from build123d import *

# Parameters (mm, degrees)
SKETCH1_W                 = 126.873
SKETCH1_H                 = 14.859
BOSS_EXTRUDE1_DEPTH       = 9.398
SKETCH2_W                 = 6.35
SKETCH2_H                 = 13.335
CUT_EXTRUDE1_DEPTH        = 128.658375969
F_5_CLEARANCE_HOLE1_D     = 3.556
F_5_CLEARANCE_HOLE1_DEPTH = 1.524
F_5_CLEARANCE_HOLE2_D     = 3.556
F_5_CLEARANCE_HOLE2_DEPTH = 14.859
F_5_CLEARANCE_HOLE3_D     = 3.556
FILLET1_R                 = 0.635


with BuildPart() as part:
    # Sketch1 → Boss-Extrude1 (new body)
    with BuildSketch(Plane(origin=(-4.699, 0, 0), x_dir=(0, -1, 0), z_dir=(-1, 0, 0))):
        with Locations((-63.4365, -5.9055)):
            Rectangle(SKETCH1_W, SKETCH1_H)
    extrude(amount=-BOSS_EXTRUDE1_DEPTH)

    # Sketch2 → Cut-Extrude1 (cut, through all)
    with BuildSketch(Plane.XZ):
        with Locations((0, -6.6675)):
            Rectangle(SKETCH2_W, SKETCH2_H)
    extrude(amount=-CUT_EXTRUDE1_DEPTH, mode=Mode.SUBTRACT)

    # #5 Clearance Hole1
    with Locations(Plane(origin=(4.699, 0, 0), x_dir=(0, 0, -1), z_dir=(1, 0, 0))):
        with Locations((8.5725, 112.3315), (8.5725, 122.1105), (8.5725, 102.5525), (8.5725, 92.7735), (8.5725, 82.9945), (8.5725, 73.2155), (8.5725, 63.4365), (8.5725, 53.6575), (8.5725, 43.8785), (8.5725, 34.0995), (8.5725, 24.3205), (8.5725, 14.5415), (8.5725, 4.7625)):
            Hole(F_5_CLEARANCE_HOLE1_D / 2, depth=F_5_CLEARANCE_HOLE1_DEPTH)

    # #5 Clearance Hole2
    with Locations(Plane.XY.offset(1.524)):
        with Locations((0, 112.3315), (0, 122.1105), (0, 102.5525), (0, 92.7735), (0, 82.9945), (0, 73.2155), (0, 63.4365), (0, 53.6575), (0, 43.8785), (0, 34.0995), (0, 24.3205), (0, 14.5415), (0, 4.7625)):
            Hole(F_5_CLEARANCE_HOLE2_D / 2, depth=F_5_CLEARANCE_HOLE2_DEPTH)

    # #5 Clearance Hole3 (through all)
    with Locations(Plane(origin=(-3.175, 0, 0), x_dir=(0, 0, -1), z_dir=(1, 0, 0))):
        with Locations((8.5725, 112.3315), (8.5725, 122.1105), (8.5725, 102.5525), (8.5725, 92.7735), (8.5725, 82.9945), (8.5725, 73.2155), (8.5725, 63.4365), (8.5725, 53.6575), (8.5725, 43.8785), (8.5725, 34.0995), (8.5725, 24.3205), (8.5725, 14.5415), (8.5725, 4.7625)):
            Hole(F_5_CLEARANCE_HOLE3_D / 2)

    # Fillet1
    fillet1_edges = [part.edges().sort_by_distance(p)[0] for p in [
        (-3.937, 126.873, -13.335),
        (-3.937, 0, -13.335),
        (3.937, 0, -13.335),
        (3.937, 126.873, -13.335),
    ]]
    fillet(fillet1_edges, radius=FILLET1_R)


solid = part.part
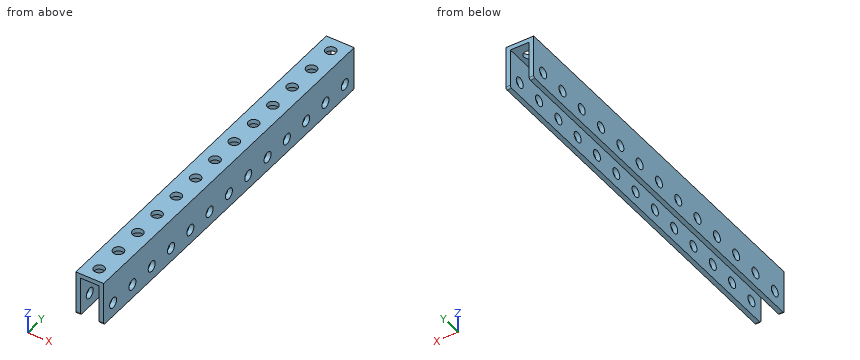
Geometry check sheet. Reference: the model listing, model coordinates, mm. Coordinates: 2 decimals unless noted, no trailing zeros. Order: outer loops, then holes, each group sorted by start corner. A loop starts at its lowest first (then second) coordinate and runs counter-clockwise, first axis right, second up. Notation, with made-up numbers: (79, 24.25) - (102, 24.25) arc R16 ccw to (102, 49.25) - close; hole circle Ø10 at (16.25, -39.5). An arc over 180 degrees is marked (long way). Answer in a Markdown table with one row per item. Add a question column.
1) Cross-section at A-A, the plane y = 49. Record the cut outline in (x, z) (3 decimals), then the cut area to 3 significant figures.
2) Material ranges on line 1 along X through (y, z) = (59, -11.5) (3 decimals); line 2 along Z through (x, y) = (-4, 64.5) (3 decimals); line 3 along Z through (x, y) = (-0.25, 36), recorded low to high. Write a range as [from, to].
3) Cross-section at B-B, the plane x = 0. State how many separate pieces and enclosed holes the cut face has, then the cut area to 3 significant figures.
4) Gauge pin test, flat ends, axial feed: P1, Ø3, axis at x = 0.5, z = -3.5, coming from the -Y side; P2, Ø4, axis at x = 0, y = 53.66, coming from the -Z side. Record the tip position at first contact, or that the pin passes through.
Check result:
| question | item | result |
|---|---|---|
| 1 | outline | (-4.699, -13.335) - (-3.175, -13.335) - (-3.175, 0) - (3.175, 0) - (3.175, -13.335) - (4.699, -13.335) - (4.699, 1.524) - (-4.699, 1.524) - close |
| 1 | area | 55.0 mm² |
| 2 | line 1 | x = [-4.699, -3.175], [3.175, 4.699] |
| 2 | line 2 | z = [-13.335, -9.997], [-7.148, 1.524] |
| 2 | line 3 | z = [0, 1.52] |
| 3 | separate pieces | 14 |
| 3 | enclosed holes | 0 |
| 3 | area | 123 mm² |
| 4 | P1 | passes through |
| 4 | P2 | stops at z = 0 |
